Answer from the drawing. Dimensions are ordinates in mm from the lowest x, y and z of the part. Round coordinates to 2 decimals unless told otherwise and drop trailing zeros. Write each loop counter-clockwise with the first axis right and the second up, starting at its lowest first coordinate (ties: lowest second). Pieces come first, ordered by that corner, then holes. Notation, with made-up numbers: M 4.25,-32 L 43.25,-32 A17 ccw 43.25,-18 Z; hole C 89,69 d8. An arc over 180 degrees is marked long. One line per item, written item: value. Start each with the question number.
(1) Consider probe 1 along Z at (x, y) = (120, 3); probe 2 along X at (y, z) = (2.05, 120.65) (3 decimals); probe 3 along Z at (x, y) = (120, 99). Determine where each line is inside the solid, lowest interval first.
(2) Section D-D (y = 12) is taken. Determine the outline of the cut face in (x, z).
(3) Given P1, Ø2, axis at x = 68.5, z = 216.5, coming from the -Y side; P2, Ø4, axis at y = 54, z = 106, coming from the +X side (3 decimals); P3, Ø8.5, axis at x = 120.65, z = 57.15, coming from the +Y side; P4, Ø5, axis at x = 89.5, z = 46, coming from the -Y side, each flat-ended and moving along its own axis, determine where each tip first touches the part or whether it passes through.
(4) Section A-A (z = 120.65) is taken. Determine the outline of the cut face in (x, y) (3 decimals).
(5) Section B-B (x = 120.65) is taken. Determine the outline of the cut face in (y, z) (3 decimals).
(6) Section C-C (y = 145.5) is taken. Determine the outline of the cut face in (x, z), plus the area to 3 significant figures.
(7) For a pull along X with two mould halves and no side action, classify the marked faces 1, 2 and 3 as released by +X, released by -X, zero draft, split by the parting line, or undercut.
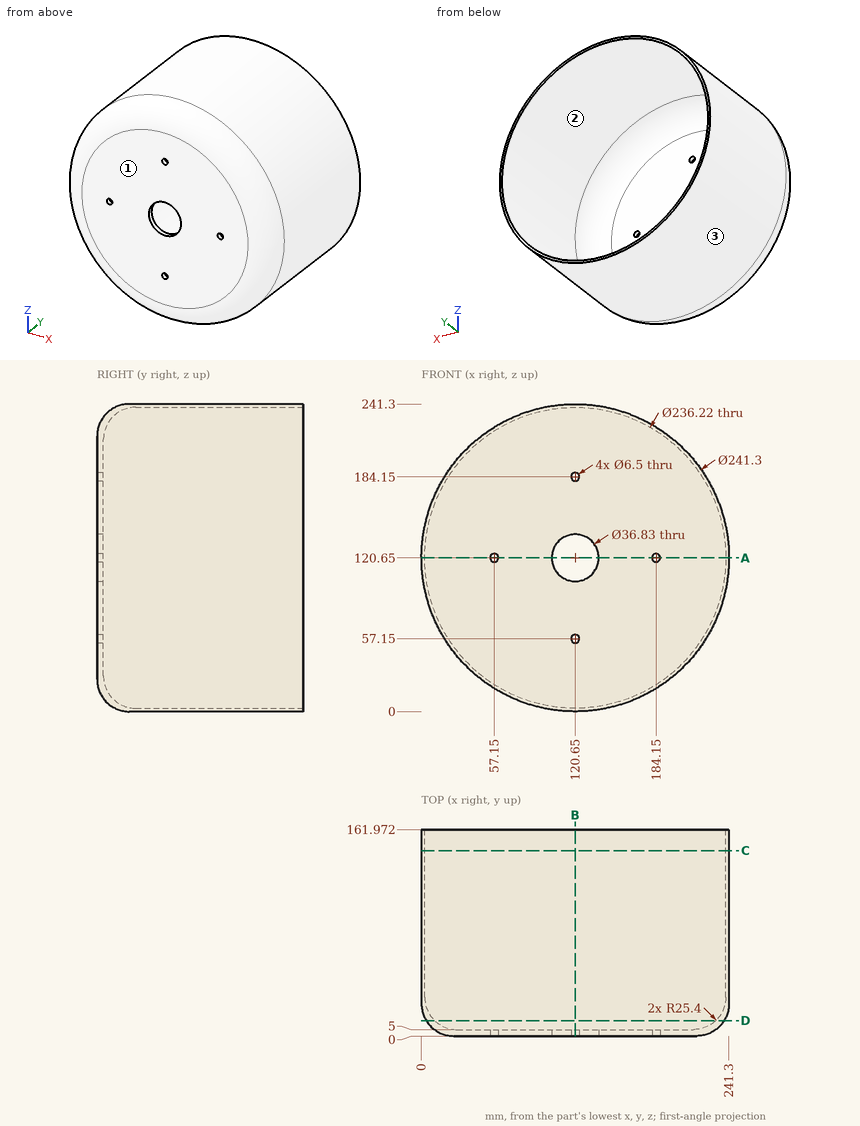
Recorded:
1. probe 1: z = 13.43 to 53.97, 60.33 to 102.25, 139.05 to 180.97, 187.33 to 227.87
1. probe 2: x = 15.403 to 53.9, 60.4 to 102.235, 139.065 to 180.9, 187.4 to 225.897
1. probe 3: z = 0 to 2.54, 238.76 to 241.3
2. outline: C 120.65,120.65 d233.66; hole C 120.65,120.65 d220.44
3. P1: stops at y = 3.5
3. P2: stops at x = 240.635
3. P3: stops at y = 5
3. P4: stops at y = 0
4. outline: M 0,25.4 A25.4 ccw 25.4,0 L 53.9,0 L 53.9,5 L 27.94,5 A25.4 cw 2.54,30.4 L 2.54,161.972 L 0,161.972 Z; M 60.4,0 L 102.235,0 L 102.235,5 L 60.4,5 Z; M 139.065,0 L 180.9,0 L 180.9,5 L 139.065,5 Z; M 187.4,0 L 215.9,0 A25.4 ccw 241.3,25.4 L 241.3,161.972 L 238.76,161.972 L 238.76,30.4 A25.4 cw 213.36,5 L 187.4,5 Z
5. outline: M 0,25.4 A25.4 ccw 25.4,0 L 161.972,0 L 161.972,2.54 L 30.4,2.54 A25.4 cw 5,27.94 L 5,53.9 L 0,53.9 Z; M 0,60.4 L 5,60.4 L 5,102.235 L 0,102.235 Z; M 0,139.065 L 5,139.065 L 5,180.9 L 0,180.9 Z; M 0,187.4 L 5,187.4 L 5,213.36 A25.4 cw 30.4,238.76 L 161.972,238.76 L 161.972,241.3 L 25.4,241.3 A25.4 ccw 0,215.9 Z
6. outline: C 120.65,120.65 d241.3; hole C 120.65,120.65 d236.22
6. area: 1,910 mm2
7. face 1: zero draft
7. face 2: undercut
7. face 3: split by the parting line
